Geometry check sheet. Reference: drawing and pictorial views, mm from the part's lowest x, y, z. A direction names the side the tool comes from. Coordinates: 2 decimals unless noted, no trailing zeros. Loops run counter-clockwise (first coordinate to the right, second up) from the corner with the lowest first, then second, coordinate; pieces in that order, holes last. Notation, with made-up numbers: (49.5, 65.5) -> (104.5, 65.5) arc R26 ccw to (104.5, 94.5) -> close; hole circle Ø1 at (-32.5, 21.5). An arc over 180 degrees is marked (long way). Answer as a JSON object with one key per item and string values. Group by question number.
Q1. Cross-section at D-D on y = 28. Record the boundary of the cut face in (x, z).
Q2. Release check for a two-part mould opening along X. For the marked faces 6, 7, 8 and 9 record: released by +X, released by -X, zero draft, split by the parting line, or undercut.
Q3. Cross-section at A-A on y = 8. Record the boundary of the cut face in (x, z) (1 decimal).
Q4. Set-up check for the marked faces 1, 2, 3, 4 and 5: record each of +Z, -Z, +X, -X, +Y, -Y from which the full face is reachable in a straight line by a thin tool's end or side.
Q5. Scan lines: L1, parallel to Y at x = 8, z = 0.3 (1 decimal); L2, parallel to Y at x = 8, z = 1.15 (1 decimal); L3, parallel to Y at x = 11.5, z = 3.9 (1 decimal). Record each from-to range of solid material in increasing order.
Q6. Cross-section at B-B on x = 8. Record the boundary of the cut face in (y, z) (1 decimal), and give its area (3 significant figures).
Q7. Cross-section at C-C on z = 3.3. Give the number of separate pieces and of enclosed holes in the cut face, and give its area (3 significant figures).
Q8. Gauge pin test, flat ends, axial feed: pin 1 Ø2.5 at (y, z) = (23, 3.5) entering from -X; pin 2 Ø9.5 at (x, y) = (9.5, 36.5) entering from -Z; pin 3 Ø1.5 at (y, z) = (17.5, 2.5) entering from +X; pin 4 Ø3 at (x, y) = (6.5, 11) entering from -Z. Record the tip position at first contact, or that the pin passes through.
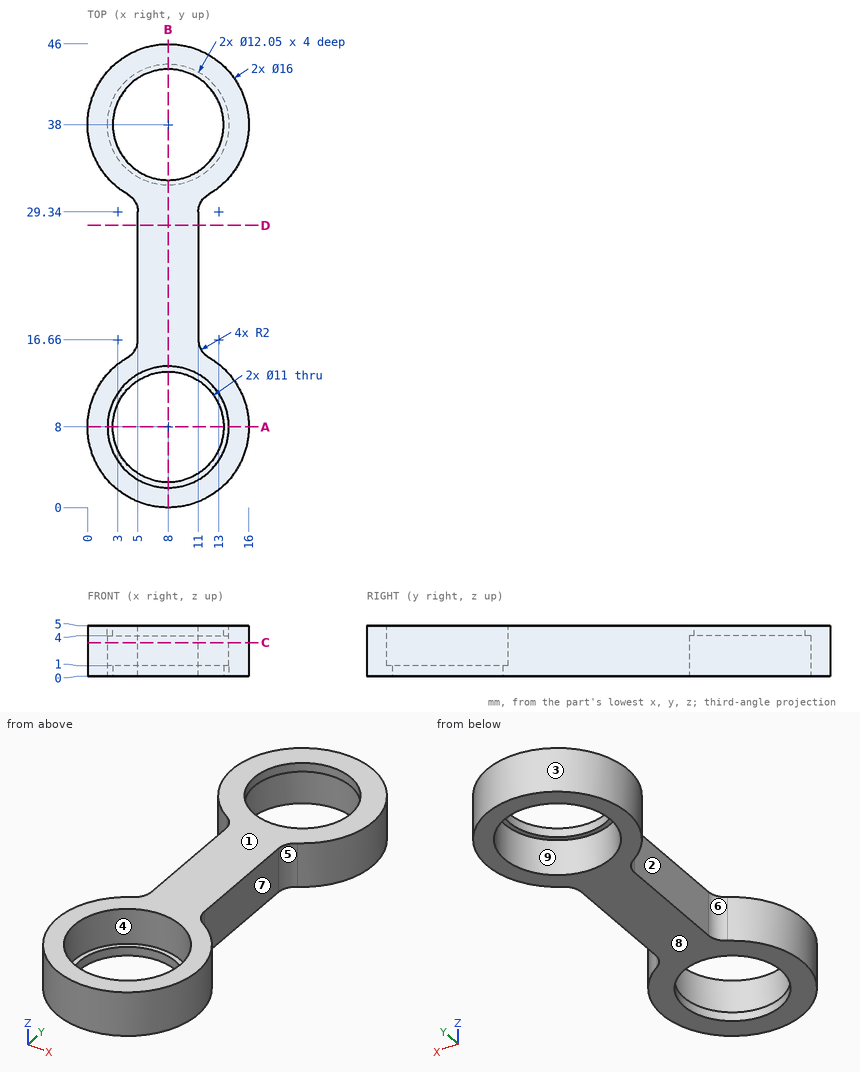
Computed values:
{
 "1": {"outline": "(5, 0) -> (11, 0) -> (11, 5) -> (5, 5) -> close"},
 "2": {"face 6": "released by -X", "face 7": "released by +X", "face 8": "zero draft", "face 9": "undercut"},
 "3": {"outline": "(0, 0) -> (2.5, 0) -> (2.5, 1) -> (2, 1) -> (2, 5) -> (0, 5) -> close; (13.5, 0) -> (16, 0) -> (16, 5) -> (14, 5) -> (14, 1) -> (13.5, 1) -> close"},
 "4": {"face 1": "+Z, +X, -X, +Y, -Y", "face 2": "+Z, -Z, -X", "face 3": "+Z, -Z", "face 4": "+Z", "face 5": "+Z, -Z, +X"},
 "5": {"L1": "y = 0 to 2.5, 13.5 to 32, 44 to 46", "L2": "y = 0 to 2, 14 to 32, 44 to 46", "L3": "y = 0.8 to 3.1, 12.9 to 15.3, 30.7 to 33.1, 42.9 to 45.2"},
 "6": {"outline": "(0, 0) -> (2.5, 0) -> (2.5, 1) -> (2, 1) -> (2, 5) -> (0, 5) -> close; (13.5, 0) -> (32, 0) -> (32, 4) -> (32.5, 4) -> (32.5, 5) -> (14, 5) -> (14, 1) -> (13.5, 1) -> close; (43.5, 4) -> (44, 4) -> (44, 0) -> (46, 0) -> (46, 5) -> (43.5, 5) -> close", "area": "112 mm²"},
 "7": {"separate pieces": "1", "enclosed holes": "2", "area": "261 mm²"},
 "8": {"pin 1": "stops at x = 5", "pin 2": "stops at z = 0", "pin 3": "stops at x = 11", "pin 4": "passes through"}
}
